Work out the finished part from the listing and answer in its coordinate system (mm). A direction names the side the tool comes from. Coordinates: 2 decimals unless noted, no trailing zeros. Order: outer loops, then holes, each group sorted by start corner. A loop starts at its lowest first (then second) coordinate and runs counter-clockwise, first axis right, second up. Notation, with made-up numbers: (23, 33.5) - (55, 33.5) arc R19 cw to (55, 54.5) - close; hole circle Ø9 at (-4.75, -21.5). An arc over 180 degrees is marked (long way). Use CSV: the item, a comma, the result in double quotes. Start each with the question number.
from build123d import *

# Parameters (mm, degrees)
SKETCH1_R           = 41
BOSS_EXTRUDE1_DEPTH = 250
CUT_EXTRUDE2_DEPTH  = 130
CUT_EXTRUDE3_DEPTH  = 205.358983849
FILLET1_R           = 5


with BuildPart() as part:
    # Sketch1 → Boss-Extrude1 (new body)
    with BuildSketch(Plane.XY):
        with BuildLine():
            Line((-100, 60), (100, 60))
            ThreePointArc((100, 60), (160, 0), (100, -60))
            Line((100, -60), (-100, -60))
            ThreePointArc((-100, -60), (-160, 0), (-100, 60))
        make_face()
        with Locations((100, 0)):
            Circle(SKETCH1_R, mode=Mode.SUBTRACT)
        with Locations(Location((-100, 0, 0), (0, 0, 180))):
            Circle(SKETCH1_R, mode=Mode.SUBTRACT)
    extrude(amount=BOSS_EXTRUDE1_DEPTH)

    # Sketch5 → Cut-Extrude2 (cut, symmetric)
    with BuildSketch(Plane(origin=(0, 0, 0), x_dir=(1, 0, 0), z_dir=(0, 1, 0))):
        Polygon((100, -215.358983849), (40, -250), (-40, -250), (-100, -215.358983849), (-160, -215.358983849), (-160, -312.331187037), (-8.326687978, -312.331187037), (8.326687978, -312.331187037), (160, -312.331187037), (160, -215.358983849), align=None)
    extrude(amount=CUT_EXTRUDE2_DEPTH, both=True, mode=Mode.SUBTRACT)

    # Sketch7 → Cut-Extrude3 (cut)
    with BuildSketch(Plane(origin=(0, 0, 0), x_dir=(-1, 0, 0), z_dir=(0, 0, -1))):
        with BuildLine():
            Line((100, 41), (5, 41))
            Line((5, 41), (5, -85.727890399))
            Line((5, -85.727890399), (141, -85.727890399))
            Line((141, -85.727890399), (141, 0))
            ThreePointArc((141, 0), (128.991378029, 28.991378029), (100, 41))
        make_face()
        with BuildLine():
            Line((-141, 0), (-141, -85.727890399))
            Line((-141, -85.727890399), (-5, -85.727890399))
            Line((-5, -85.727890399), (-5, 41))
            Line((-5, 41), (-100, 41))
            ThreePointArc((-100, 41), (-128.991378029, 28.991378029), (-141, 0))
        make_face()
    extrude(amount=-CUT_EXTRUDE3_DEPTH, mode=Mode.SUBTRACT)

    # Fillet1
    fillet1_edges = [part.edges().sort_by_distance(p)[0] for p in [
        (5, -9.5, 205.358983849),
        (5, 41, 102.679491924),
        (-5, -9.5, 205.358983849),
        (-5, 41, 102.679491924),
    ]]
    fillet(fillet1_edges, radius=FILLET1_R)


solid = part.part
1) Straight lines are drawn through the part: line 1 (X direction, y = 0, z = 84.5); line 2 (X direction, y = 32, z = 152.5); line 3 (X direction, y = -52, z = 96.5). For each, find the intervals that lie inside material, in ascending order. Write a range as [from, to].
2) The part is cut by section C-C on z = 102. Determine the outline of the cut face in (x, y), plus the area to 3 significant figures.
3) Flat-ended cylindrical pins translate along their axes: P1, Ø2, axis at y = 7.5, z = 127, coming from the -X side; P2, Ø4, axis at y = 32.5, z = 196.5, coming from the -X side; P3, Ø5, axis at y = -37, z = 29.5, coming from the -X side. Find the tip coordinate at first contact, or state that the pin passes through.
4) The part is cut by section B-B on z = 210. Determine the outline of the cut face in (x, y), plus the area to 3 significant figures.
5) The part is cut by section A-A on y = 17. Determine the outline of the cut face in (x, z), plus the area to 3 significant figures.
6) The part is cut by section D-D on x = 66.5. Determine the outline of the cut face in (y, z), plus the area to 3 significant figures.
7) For faces 4 (the face through (144, 1, 215.359)), 5 (the face through (-143, 1, 215.359)), 6 (the face through (121.02, 35.2, 145.9)), 7 (the face through (-5, -11, 99)), 8 (the face through (-1, 60, 123)), determine the directions among +Z, -Z, +X, -X, +Y, -Y from which every point of the face is accessible in a straight line to the end or side of a thin tool.
8) For a pull along Y with two mould halves and no side action, classify faces 1 (the face through (-56.25, 0.84, 240.62)), 2 (the face through (-56, 41, 101)), 3 (the face through (-127.7, 30.23, 137.03)) as +Y half, -Y half, draft (parallel to the pull), parting line (faces both ways), or undercut.
Answer key:
1,line 1,"[-160, -141], [-5, 5], [141, 160]"
1,line 2,"[-150.75, -125.63], [-5, 5], [125.63, 150.75]"
1,line 3,"[-5, 5]"
2,outline,"(-141, -43.81) - (-141, 0) arc R41 cw to (-100, 41) - (-10, 41) arc R5 cw to (-5, 36) - (-5, -60) - (5, -60) - (5, 36) arc R5 cw to (10, 41) - (100, 41) arc R41 cw to (141, 0) - (141, -43.81) arc R60 ccw to (100, 60) - (-100, 60) arc R60 ccw to start"
2,area,"8,990 mm^2"
3,P1,"x = -159.65"
3,P2,"x = -151.67"
3,P3,"x = -149.09"
4,outline,"(-100, -60) - (100, -60) arc R60 ccw to (100, 60) - (-100, 60) arc R60 ccw to start; hole circle Ø82 at (-100, 0); hole circle Ø82 at (100, 0)"
4,area,"24,700 mm^2"
5,outline,"(-157.54, 0) - (-137.31, 0) - (-137.31, 215.36) - (-157.54, 215.36) - close; (-62.69, 205.36) - (-10, 205.36) arc R5 cw to (-5, 200.36) - (-5, 0) - (5, 0) - (5, 200.36) arc R5 cw to (10, 205.36) - (62.69, 205.36) - (62.69, 236.9) - (40, 250) - (-40, 250) - (-62.69, 236.9) - close; (137.31, 0) - (157.54, 0) - (157.54, 215.36) - (137.31, 215.36) - close"
5,area,"16,100 mm^2"
6,outline,"(-60, 205.36) - (-23.64, 205.36) - (-23.64, 234.7) - (-60, 234.7) - close; (23.64, 205.36) - (41, 205.36) - (41, 0) - (60, 0) - (60, 234.7) - (23.64, 234.7) - close"
6,area,"6,040 mm^2"
7,face 4,"+Z, +X, +Y, -Y"
7,face 5,"+Z, -X, +Y, -Y"
7,face 6,"+Z, -Z"
7,face 7,"-Z, -Y"
7,face 8,"+Z, -Z, +X, -X, +Y"
8,face 1,"draft"
8,face 2,"-Y half"
8,face 3,"undercut"
